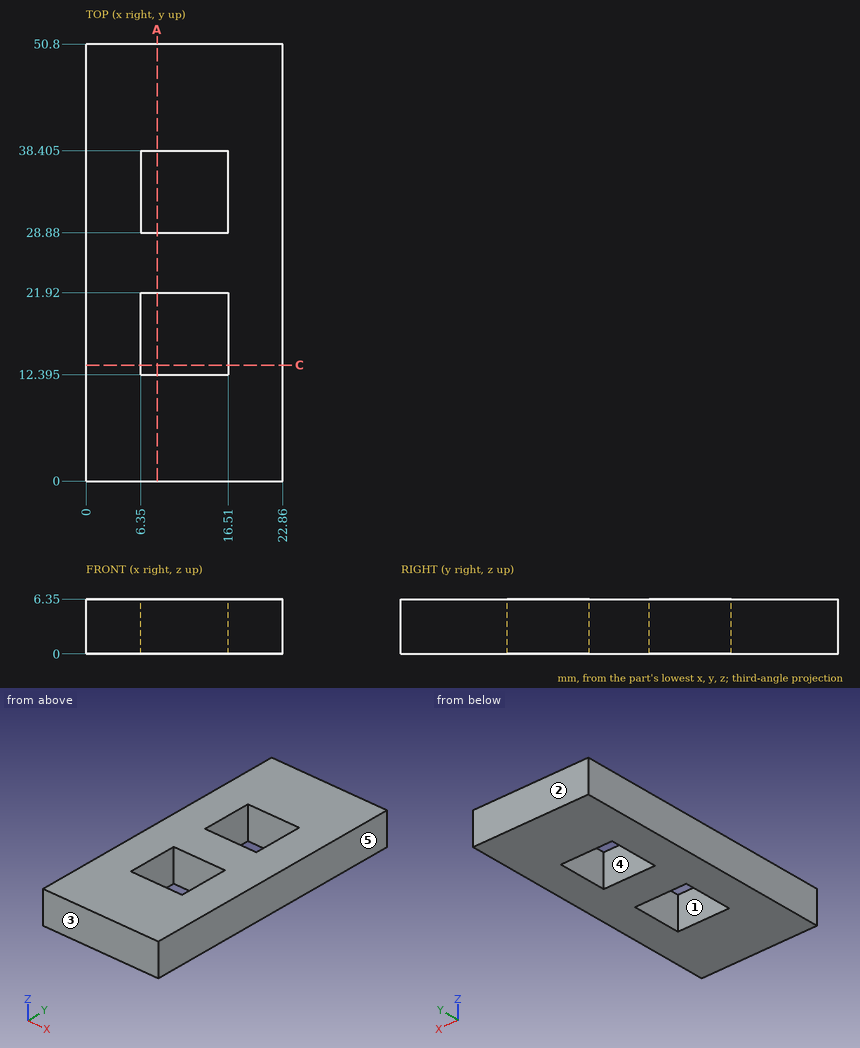
Can you work these out from the drawing? Everything is in mm from the part's minimum corner. A direction names the side the tool comes from. Coordinates: 2 decimals unless noted, no trailing zeros. Loops run counter-clockwise (first coordinate to the right, second up) from the corner with the lowest first, then second, coordinate; pieces in that order, holes last.
1. Imagine slicing it at A-A, the plane x = 8.25. Count the separate pieces of the cut face and the enclosed holes in it, and give its area (3 significant figures).
2. For P1, Ø1.9, axis at x = 10.5, z = 4.5, coming from the -Y side, with a flat end and sliding along its axis, tell me the tip position at first contact or that it passes through.
3. Imagine slicing it at C-C, the plane y = 13.5. Please give me the cut outline in (x, z).
4. If we mould it in two halves opening along X, with no side actions, what happens to the marked faces 3, 4 and 5? For each: pulls with the +X half, pulls with the -X half, needs draft (parallel to the pull), parting line crosses it, or undercut.
5. For the marked faces 1 and 2, which set-ups out of +Z, -Z, +X, -X, +Y, -Y let a thin tool reach every point of the face, with its end or its side?
6. I need wall thicknesses on L1, parallel to Y at x = 9.25, z = 0.75 (1 decimal); L2, parallel to X at y = 16.5, z = 3.75. Which ranges of each line are inside material? Lowest first, please.
Taken from the geometry:
1. separate pieces: 3
1. enclosed holes: 0
1. area: 202 mm2
2. P1: stops at y = 0
3. outline: (0, 0) - (6.35, 0) - (6.35, 6.35) - (0, 6.35) - close; (16.51, 0) - (22.86, 0) - (22.86, 6.35) - (16.51, 6.35) - close
4. face 3: needs draft
4. face 4: undercut
4. face 5: pulls with the +X half
5. face 1: +Z, -Z
5. face 2: +Z, -Z, +X, -X, +Y
6. L1: y = 0 to 12.4, 21.9 to 28.9, 38.4 to 50.8
6. L2: x = 0 to 6.35, 16.51 to 22.86
